Model file for the job. Use its own axes, mm. A direction names the side the tool comes from. Give positions to 0.01 mm unless a question says otherwise; leave off trailing zeros. Loops run counter-clockwise (first coordinate to the right, second up) from the corner with the lowest first, then second, coordinate; pieces in that order, holes last. Notation, with made-up numbers: (5.25, -10) -> (25.25, -10) arc R7 ccw to (25.25, -6) -> close; hole circle Ø7 at (-1.75, -26.5). An arc over 180 degrees is marked (long way). Use CSV: the item, a comma, the result in double quotes. Start each with the question number.
(1) Cut at B-B on z = -41.5. Write the cut outline in (x, y).
(2) 3-axis set-ups, long thin cutter, end or side, ignore diameter. For faces 5 (the flat face through (-25, 7.5, 43)), 6 (the flat face through (-26, 11.636, -42)), 7 (the flat face through (0, 9, 35)), 8 (the flat face through (0, 10, 37)): which of +Z, -Z, +X, -X, +Y, -Y reach the whole face in a straight line?
(3) Pull direction X, two halves, no side cores. Call faces 1 (the flat face through (28, 18, -8)), 2 (the cylindrical face through (24.232, 29.072, -47.432)), 3 (the flat face through (22, 20, 46)), 4 (the flat face through (-25, 32.5, 43)): pulls with the +X half, pulls with the -X half, needs draft (parallel to the pull), parting line crosses it, or undercut.
(4) Drill centre lines: probe 1 along X at (y, z) = (34, -30.5); probe 2 along X at (y, z) = (28.5, 39); probe 3 along Y at (x, z) = (8, -12). Where is each one in solid material? Low to high.
(5) Cut at A-A on x = 3.5. Write the cut outline in (y, z).
(6) Cut at C-C on z = -7.5. Write the cut outline in (x, y), then the cut area to 3 significant figures.
(7) Flat gauge pins, fed straight in: pin 1 (7.5 mm diameter, centred on y = 16, z = 47, fed in from +X); pin 2 (5 mm diameter, centred on x = -12, y = 11, fed in from -Z); pin 3 (4 mm diameter, centred on x = -16, y = 7, fed in from -Z). Where does each tip first touch, or does it go through?
from build123d import *

# Parameters (mm, degrees)
SKETCH1_W           = 50
SKETCH1_H           = 70
BOSS_EXTRUDE1_DEPTH = 40
SHELL1_T            = 3
BOSS_EXTRUDE2_START = -2
BOSS_EXTRUDE2_DEPTH = 5
CUT_EXTRUDE1_DEPTH  = 87.984136485
BOSS_EXTRUDE4_DEPTH = 5
SKETCH8_R           = 7.5
CUT_EXTRUDE2_DEPTH  = 2.5
SKETCH9_W           = 40
SKETCH9_H           = 30
CUT_EXTRUDE3_DEPTH  = 10
CUT_EXTRUDE4_DEPTH  = 10


with BuildPart() as part:
    # Sketch1 → Boss-Extrude1 (new body)
    with BuildSketch(Plane(origin=(0, 0, 0), x_dir=(1, 0, 0), z_dir=(0, 1, 0))):
        Rectangle(SKETCH1_W, SKETCH1_H)
    extrude(amount=BOSS_EXTRUDE1_DEPTH)

    # Shell1
    shell1_openings = [part.faces().sort_by_distance(p)[0] for p in [
        (0, 40, 0),
    ]]
    offset(amount=SHELL1_T, openings=shell1_openings, kind=Kind.INTERSECTION)

    # Sketch2 → Boss-Extrude2 (add)
    with BuildSketch(Plane.ZY.offset(-25).offset(BOSS_EXTRUDE2_START)):
        with BuildLine():
            Line((38, 32.5), (48, 32.5))
            ThreePointArc((48, 32.5), (53.2, 20), (48, 7.5))
            Line((48, 7.5), (38, 7.5))
            Line((38, 7.5), (38, 32.5))
        make_face()
    boss_extrude2 = extrude(amount=BOSS_EXTRUDE2_DEPTH)

    # Mirror1: Boss-Extrude2 across plane
    add(boss_extrude2.mirror(Plane.ZY))

    # Sketch4 → Cut-Extrude1 (cut, through all)
    with BuildSketch(Plane.ZY.offset(28)):
        Polygon((-38, 40), (38, 40), (38, 32.5), align=None)
    extrude(amount=-CUT_EXTRUDE1_DEPTH, mode=Mode.SUBTRACT)

    # Sketch7 → Boss-Extrude4 (add)
    with BuildSketch(Plane.ZY.offset(28)):
        with BuildLine():
            Line((-38, 31.635993136), (-45.5, 31.635993136))
            ThreePointArc((-45.5, 31.635993136), (-55.5, 21.635993136), (-45.5, 11.635993136))
            Line((-45.5, 11.635993136), (-38, 11.635993136))
            Line((-38, 11.635993136), (-38, 31.635993136))
        make_face()
    boss_extrude4 = extrude(amount=-BOSS_EXTRUDE4_DEPTH)

    # Mirror3: Boss-Extrude4 across plane
    add(boss_extrude4.mirror(Plane.ZY))

    # Sketch8 → Cut-Extrude2 (cut)
    with BuildSketch(Plane.ZY.offset(-23)):
        with Locations((-46.455887692, 21.635993136)):
            Circle(SKETCH8_R)
    cut_extrude2 = extrude(amount=-CUT_EXTRUDE2_DEPTH, mode=Mode.SUBTRACT)

    # Mirror4: Cut-Extrude2 across plane
    add(cut_extrude2.mirror(Plane.ZY), mode=Mode.SUBTRACT)

    # Sketch9 → Cut-Extrude3 (cut)
    with BuildSketch(Plane(origin=(0, 0, -38), x_dir=(-1, 0, 0), z_dir=(0, 0, -1))):
        with Locations((0, 21.635993136)):
            Rectangle(SKETCH9_W, SKETCH9_H)
    extrude(amount=-CUT_EXTRUDE3_DEPTH, mode=Mode.SUBTRACT)

    # 3DSketch1 → Cut-Extrude4 (cut)
    with BuildSketch(Plane(origin=(20, 10, 38), x_dir=(-0.894427190999916, 0.447213595499958, 0), z_dir=(0, 0, 1))):
        Polygon((0, 0), (35.77708764, 17.88854382), (44.72135955, 0), (8.94427191, -17.88854382), align=None)
    extrude(amount=-CUT_EXTRUDE4_DEPTH, mode=Mode.SUBTRACT)


solid = part.part
Check result:
1,outline,"(-28, 11.64) -> (-23, 11.64) -> (-23, 16.01) -> (-25.5, 16.01) -> (-25.5, 27.27) -> (-23, 27.27) -> (-23, 31.64) -> (-28, 31.64) -> close; (23, 11.64) -> (28, 11.64) -> (28, 31.64) -> (23, 31.64) -> (23, 27.27) -> (25.5, 27.27) -> (25.5, 16.01) -> (23, 16.01) -> close"
2,face 5,"+Z, +X, -X, -Y"
2,face 6,"-Z, +X, -X, -Y"
2,face 7,"+Y"
2,face 8,"+Z, -Z"
3,face 1,"pulls with the +X half"
3,face 2,"undercut"
3,face 3,"undercut"
3,face 4,"needs draft"
4,probe 1,"-28 to -25, 25 to 28"
4,probe 2,"-27 to -22, 22 to 27"
4,probe 3,"-3 to 0"
5,outline,"(-3, -38) -> (6.64, -38) -> (6.64, -35) -> (0, -35) -> (0, 35) -> (10, 35) -> (10, 38) -> (-3, 38) -> close; (30, 35) -> (32.8, 35) -> (32.5, 38) -> (30, 38) -> close; (36.64, -38) -> (40, -38) -> (39.7, -35) -> (36.64, -35) -> close"
6,outline,"(-28, -3) -> (28, -3) -> (28, 36.99) -> (25, 36.99) -> (25, 0) -> (-25, 0) -> (-25, 36.99) -> (-28, 36.99) -> close"
6,area,"390 mm²"
7,pin 1,"x = 27"
7,pin 2,"z = 35"
7,pin 3,"z = -38"
